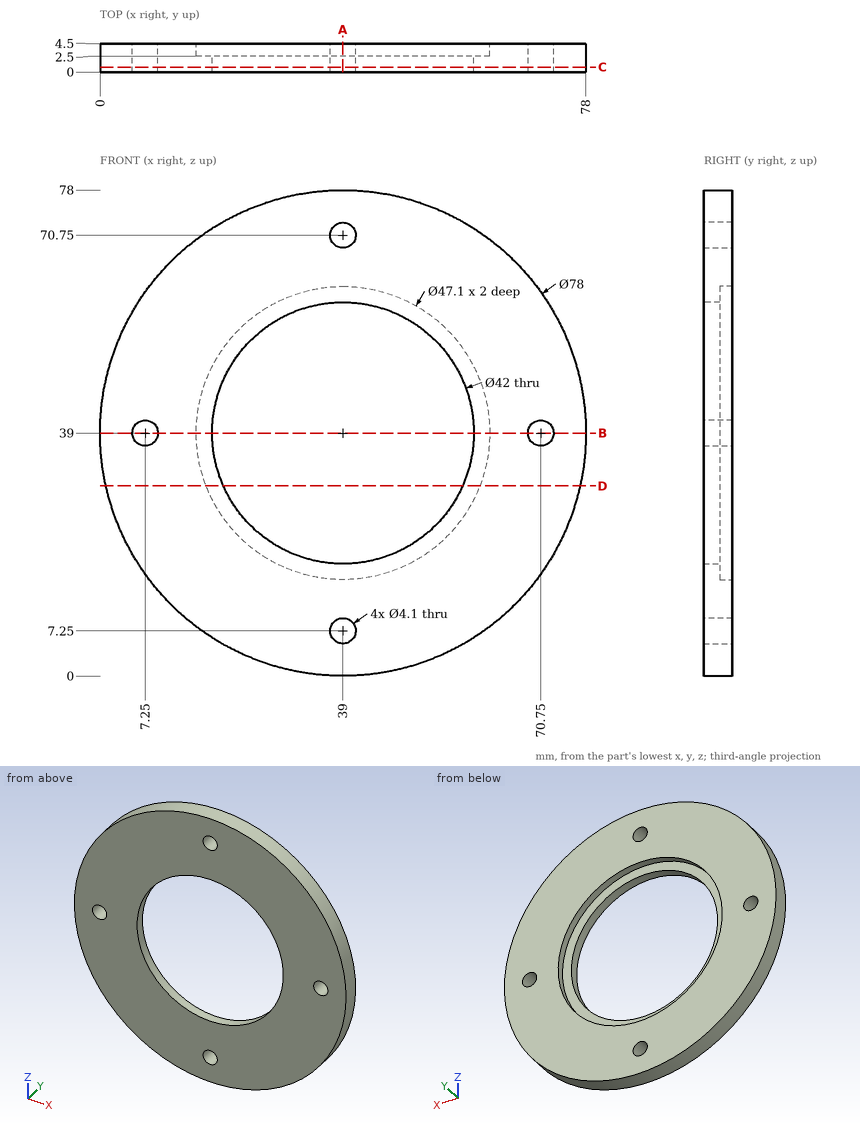
Job drawing, mm, ordinate dimensions from the low corner. One solid piece. Coordinates: 2 decimals unless noted, no trailing zeros. Write each loop counter-clockwise with the first axis right and the second up, starting at its lowest first coordinate (ties: lowest second). Pieces come first, ordered by that corner, then holes.
Item 1: Slice it at B-B (z = 39). Write the cut outline in (x, y), and give its area (3 significant figures).
Item 2: Pin check, flat tips, straight feed: pin 1 (1.5 mm diameter, centred on x = 67.5, y = 2, fed in from -Z); pin 2 (1.5 mm diameter, centred on x = 24, y = 2, fed in from -Z); pin 3 (4.5 mm diameter, centred on x = 7.25, z = 39, fed in from -Y); pin 4 (23.5 mm diameter, centred on x = 35.5, z = 48.5, fed in from +Y). Stop position of each tip, or through.
Item 3: Slice it at C-C (y = 0.8). Write the cut outline in (x, z), and give its area (3 significant figures).
Item 4: Slice it at D-D (z = 30.5). Write the cut outline in (x, y).
Item 5: Probe line 1 (X direction, y = 1.55, z = 39); line 2 (X direction, y = 3.15, z = 39); line 3 (Z direction, x = 31, y = 1.9). List the from-to ranges inside material, lowest first.
Item 6: Slice it at A-A (x = 39). Write the cut outline in (y, z).
Results found:
1. outline: (0, 0) - (5.2, 0) - (5.2, 4.5) - (0, 4.5) - close; (9.3, 0) - (18, 0) - (18, 2.5) - (15.45, 2.5) - (15.45, 4.5) - (9.3, 4.5) - close; (60, 0) - (68.7, 0) - (68.7, 4.5) - (62.55, 4.5) - (62.55, 2.5) - (60, 2.5) - close; (72.8, 0) - (78, 0) - (78, 4.5) - (72.8, 4.5) - close
1. area: 115 mm2
2. pin 1: stops at z = 11.6
2. pin 2: stops at z = 2.7
2. pin 3: stops at y = 0
2. pin 4: stops at y = 2.5
3. outline: circle Ø78 at (39, 39); hole circle Ø4.1 at (7.25, 39); hole circle Ø42 at (39, 39); hole circle Ø4.1 at (39, 7.25); hole circle Ø4.1 at (39, 70.75); hole circle Ø4.1 at (70.75, 39)
3. area: 3,340 mm2
4. outline: (0.94, 0) - (19.8, 0) - (19.8, 2.5) - (17.04, 2.5) - (17.04, 4.5) - (0.94, 4.5) - close; (58.2, 0) - (77.06, 0) - (77.06, 4.5) - (60.96, 4.5) - (60.96, 2.5) - (58.2, 2.5) - close
5. line 1: x = 0 to 5.2, 9.3 to 18, 60 to 68.7, 72.8 to 78
5. line 2: x = 0 to 5.2, 9.3 to 15.45, 62.55 to 68.7, 72.8 to 78
5. line 3: z = 0.83 to 19.58, 58.42 to 77.17
6. outline: (0, 0) - (4.5, 0) - (4.5, 5.2) - (0, 5.2) - close; (0, 9.3) - (4.5, 9.3) - (4.5, 15.45) - (2.5, 15.45) - (2.5, 18) - (0, 18) - close; (0, 60) - (2.5, 60) - (2.5, 62.55) - (4.5, 62.55) - (4.5, 68.7) - (0, 68.7) - close; (0, 72.8) - (4.5, 72.8) - (4.5, 78) - (0, 78) - close
